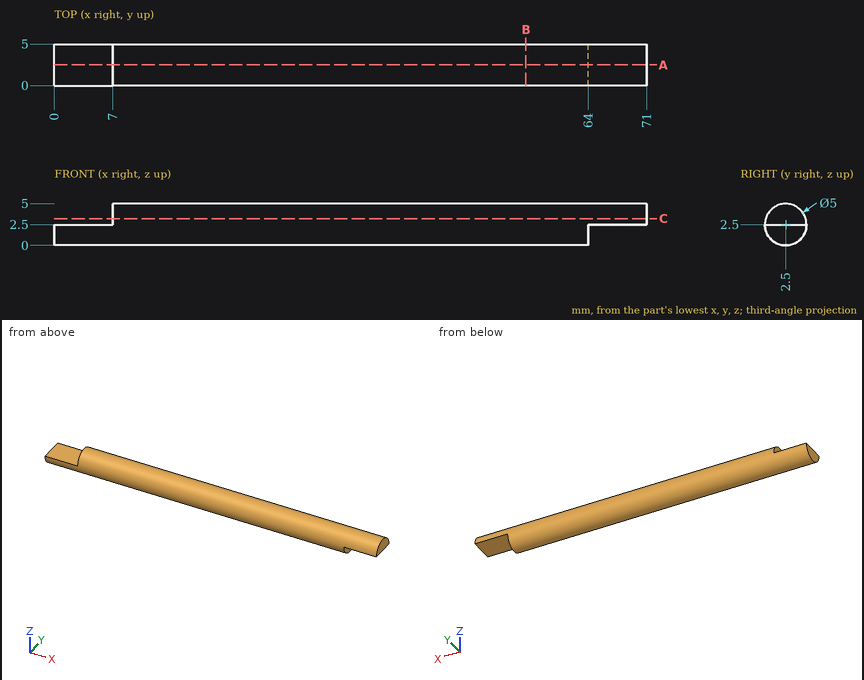
Source: three-view drawing plus pictorial views. Frame: mm from the lowest corner of the part. Round coordinates to 2 decimals unless told otherwise and drop trailing zeros. Loops run counter-clockwise (first coordinate to the right, second up) from the corner with the lowest first, then second, coordinate; pieces in that order, holes last.
1. Contact query for flat-ended pins moving along their axis: pin 1 (3 mm diameter, centred on y = 2, z = 1.5, fed in from +X); pin 2 (1.5 mm diameter, centred on x = 2.5, y = 3, fed in from +Z). Output: stop coordinate, or through.
2. Section query C-C on z = 3.2. Output: boundary loops of the cut face in (x, y), and give its area (3 significant figures).
3. Section query B-B on x = 56.5. Output: boundary loops of the cut face in (y, z), and give its area (3 significant figures).
4. Ray query, L1, parallel to X at y = 4.65, z = 2.9; L2, parallel to X at y = 3.7, z = 2.05; L3, parallel to Y at x = 5, z = 0.65. Return the intervals inside material, ascending.
5. Section query A-A on y = 2.5. Output: boundary loops of the cut face in (x, z), and give its area (3 significant figures).
Answers below:
1. pin 1: stops at x = 71
1. pin 2: stops at z = 2.5
2. outline: (7, 0.1) - (71, 0.1) - (71, 4.9) - (7, 4.9) - close
2. area: 307 mm2
3. outline: circle Ø5 at (2.5, 2.5)
3. area: 19.6 mm2
4. L1: x = 7 to 71
4. L2: x = 0 to 64
4. L3: y = 0.82 to 4.18
5. outline: (0, 0) - (64, 0) - (64, 2.5) - (71, 2.5) - (71, 5) - (7, 5) - (7, 2.5) - (0, 2.5) - close
5. area: 320 mm2
